Autodesk Inventor part; units mm, degrees
ref_plane "YZ Plane" through (0, 0, 0) normal (1, 0, 0) x (0, 1, 0)
ref_plane "XZ Plane" through (0, 0, 0) normal (0, 1, 0) x (-1, 0, 0)
ref_plane "XY Plane" through (0, 0, 0) normal (0, 0, 1) x (1, 0, 0)
sketch "Sketch4" plane through (0, 0, 0) normal (0, 1, 0) x (-1, 0, 0)
  circle A0 centre (-1.9122, 1.2943) radius 36.25
  circle A1 centre (0, 0) radius 45.5
  circle A2 centre (41.25, 0) radius 2.05
  circle A3 centre (0, 41.25) radius 2.05
  circle A4 centre (-41.25, 0) radius 2.05
  circle A5 centre (0, -41.25) radius 2.05
  dimension "d18" = 91
  dimension "d20" = 4.1
  dimension "d23" = 360
extrude "Extrusion4" add sketch "Sketch4" along normal blind 2.5 contours A0 | A1
sketch "Sketch5" plane through (0, 0, 0) normal (0, -1, 0) x (1, 0, 0)
  circle A0 centre (-41.25, 0) radius 2.05
  circle A1 centre (0, 41.25) radius 2.05
  circle A2 centre (41.25, 0) radius 2.05
  circle A3 centre (0, -41.25) radius 2.05
  circle A4 centre (-41.25, 0) radius 3
  circle A5 centre (0, 41.25) radius 3
  circle A6 centre (41.25, 0) radius 3
  circle A7 centre (0, -41.25) radius 3
  point P0 (0, 0)
  dimension "d27" = 6
  dimension "d28" = 6
  dimension "d29" = 6
  dimension "d30" = 6
extrude "Extrusion5" cut sketch "Sketch5" against normal blind 1.25 contours A0 | A1 | A2 | A3 | A4 | A5 | A6 | A7
fillet "Fillet2" radius 1 2 edges at (45.5, 0, 0) (45.5, 2.5, 0)
properties part number "Base_Cover" material "Acetal Resin, White"
Can you work these out from the model? Positions are in its coordinate system, mm. A direction names the side the tool comes from. Round coordinates to 2 decimals unless told otherwise and drop trailing zeros. Loops run counter-clockwise (first coordinate to the right, second up) from the corner with the lowest first, then second, coordinate; pieces in that order, holes last. Notation, with made-up numbers: M -20.5,38 L -12.5,38 A21 ccw -12.5,49 Z; hole C 32,-40 d3. An arc over 180 degrees is marked long. Write item = value, one per line. Start each with the question number.
(1) Which directions (+Z, -Z, +X, -X, +Y, -Y) give clear straight access to the entire face, cutting with the end or side of a thin tool? Please do faces 1 (the face through (0.267, 1.866, 39.217)), 2 (the face through (-0.391, 0.616, -38.276)).
(2) Suppose I cut it at B-B on y = 0.4. Write out the boundary of the cut face in (x, z), plus the area to 3 significant figures.
(3) I need wall thicknesses on line 1 along Z through (x, y) = (-0.5, 0.45); line 2 along Z through (x, y) = (1.5, 2); line 3 along X through (y, z) = (2, 41.25). Which ranges of each line are inside material? Lowest first, please.
(4) If we mould it in two halves opening along X, with no side actions, what happens to faces 3 (the face through (1, 0, 1)), 4 (the face through (36.107, 1.246, 27.686)), 5 (the face through (-44.247, 0.616, 0.132))? For each: released by +X, released by -X, zero draft, split by the parting line, or undercut.
(5) Suppose I cut it at A-A on x = 0. Write out the boundary of the cut face in (y, z), plus the area to 3 significant figures.
(6) I'm going to push flat-ended pins straight in: P1, Ø1.8, axis at x = -1, z = 40, coming from the -Y side; P2, Ø1, axis at y = 1.5, z = -25, coming from the -X side; P3, Ø3.5, axis at x = -41.25, z = 0, coming from the -Y side; P4, Ø8, axis at x = 0, z = 41.25, coming from the +Y side. Where does each tip first touch, or does it pass through?
Answer block:
q1.face_1 = +Y, -Y
q1.face_2 = -Y
q2.outline = C 0,0 d90.6; hole C -41.25,0 d6; hole C 0,-41.25 d6; hole C 0,41.25 d6; hole C 41.25,0 d6
q2.area = 6,330 mm²
q3.line_1 = -45.33 to -44.21, -38.29 to 38.29, 44.21 to 45.33
q3.line_2 = -45.34 to -42.65, -39.85 to 39.85, 42.65 to 45.34
q3.line_3 = -18.88 to -2.05, 2.05 to 18.88
q4.face_3 = zero draft
q4.face_4 = split by the parting line
q4.face_5 = undercut
q5.outline = M 0,-44.5 A1 ccw 1,-45.5 L 1.5,-45.5 A1 ccw 2.5,-44.5 L 2.5,-43.3 L 1.25,-43.3 L 1.25,-44.25 L 0,-44.25 Z; M 0,-38.25 L 1.25,-38.25 L 1.25,-39.2 L 2.5,-39.2 L 2.5,39.2 L 1.25,39.2 L 1.25,38.25 L 0,38.25 Z; M 0,44.25 L 1.25,44.25 L 1.25,43.3 L 2.5,43.3 L 2.5,44.5 A1 ccw 1.5,45.5 L 1,45.5 A1 ccw 0,44.5 Z
q5.area = 201 mm²
q6.P1 = 1.25
q6.P2 = -38.34
q6.P3 = through
q6.P4 = 2.5
